```python
from build123d import *

# Parameters (mm, degrees)
SKETCH1_R               = 4.5
BOSS_EXTRUDE1_DEPTH     = 144
CUT_EXTRUDE1_START      = -3
SKETCH3_W               = 8
SKETCH3_H               = 9
CUT_EXTRUDE1_DEPTH      = 1.5
FILLET1_R               = 0.75
CUT_EXTRUDE2_DEPTH      = 145.265380565
CUT_EXTRUDE2_DEPTH_BACK = 145.265380565
SKETCH4_R               = 2.125


with BuildPart() as part:
    # Sketch1 → Boss-Extrude1 (new body)
    with BuildSketch(Plane.XY):
        Circle(SKETCH1_R)
    extrude(amount=BOSS_EXTRUDE1_DEPTH)

    # Sketch3 → Cut-Extrude1 (cut)
    with BuildSketch(Plane(origin=(0, 0, 0), x_dir=(0, 0, -1), z_dir=(1, 0, 0)).offset(CUT_EXTRUDE1_START)):
        with Locations((-140, 0)):
            Rectangle(SKETCH3_W, SKETCH3_H)
    cut_extrude1 = extrude(amount=-CUT_EXTRUDE1_DEPTH, mode=Mode.SUBTRACT)

    # Mirror1: Cut-Extrude1 across plane
    add(cut_extrude1.mirror(Plane(origin=(0, 0, 0), x_dir=(0, 0, 1), z_dir=(1, 0, 0))), mode=Mode.SUBTRACT)

    # Fillet1
    fillet1_edges = [part.edges().sort_by_distance(p)[0] for p in [
        (0, 4.5, 144),
        (0, -4.5, 144),
    ]]
    fillet(fillet1_edges, radius=FILLET1_R)

    # Sketch4 → Cut-Extrude2 (cut, two sides: drawn at the far end of the back side and taken through both)
    with BuildSketch(Plane(origin=(3, 0, 0), x_dir=(0, 0, -1), z_dir=(1, 0, 0)).offset(-CUT_EXTRUDE2_DEPTH_BACK)):
        with Locations((-140, 0.354101966)):
            Circle(SKETCH4_R)
    extrude(amount=CUT_EXTRUDE2_DEPTH + CUT_EXTRUDE2_DEPTH_BACK, mode=Mode.SUBTRACT)


solid = part.part
```
Geometry: final body of the model. Coordinates: model frame, mm. A direction names the side the tool comes from. Round coordinates to 2 decimals unless told otherwise and drop trailing zeros. Order: outer loops, then holes, each group sorted by start corner. A loop starts at its lowest first (then second) coordinate and runs counter-clockwise, first axis right, second up. Notation, with made-up numbers: M 84.25,88 L 105.25,88 A12 cw 105.25,100 Z; hole C 50,76.5 d4. An arc over 180 degrees is marked long. One line per item, written item: value.
(1) Pull-direction query (Z, two-part tool) for faces 1 (the flat face through (0, 0, 144)), 2 (the cylindrical face through (-0.042, 0.448, 142.123)), 3 (the flat face through (0, 0, 0)), 4 (the flat face through (3, -2, 140)); classes: pulls with the +Z half, pulls with the -Z half, needs draft (parallel to the pull), parting line crosses it, or undercut.
Result sheet:
face 1: pulls with the +Z half
face 2: undercut
face 3: pulls with the -Z half
face 4: needs draft
(2) Pin query (flat end, axial travel): P1, Ø0.8, axis at x = -4, y = 1, coming from the +Z side; P2, Ø1, axis at x = 1.5, z = 109, coming from the +Y side; P3, Ø3.5, axis at y = 1.5, z = 140, coming from the -X side; P4, Ø1.6, axis at x = 3.5, y = 1, coming from the +Z side. Return the tip coordinate at first contact, or that it passes through.
Result sheet:
P1: z = 136
P2: y = 4.39
P3: x = -3
P4: z = 144
(3) Cut plane A-A (z = 140). Return the cut outline in (x, y).
Result sheet:
outline: M -3,-3.35 A4.5 ccw 3,-3.35 L 3,-1.77 L -3,-1.77 Z; M -3,2.48 L 3,2.48 L 3,3.35 A4.5 ccw -3,3.35 Z
(4) Line query: probe 1 along Z at (x, y) = (2.5, 0.5); probe 2 along Y at (x, z) = (0.5, 28); probe 3 along Y at (x, z) = (0.05, 140). Output: solid intervals per line, ascending. Write a range as [from, to].
Result sheet:
probe 1: [0, 137.88], [142.12, 144]
probe 2: [-4.47, 4.47]
probe 3: [-4.5, -1.77], [2.48, 4.5]
(5) Reachability of faces 5 (the flat face through (-3, -2, 140)), 6 (the cylindrical face through (-0.59, 4.46, 70.62)) from +Z, -Z, +X, -X, +Y, -Y: full face, straight path, thin tool, end or side. Return the list, or none.
Result sheet:
face 5: +Z, -X, +Y, -Y
face 6: +Z, -Z
(6) Cut plane B-B (z = 77.5). Return the cut outline in (x, y), and give its area (3 significant figures).
Result sheet:
outline: C 0,0 d9
area: 63.6 mm2
